```python
from build123d import *

# Parameters (mm, degrees)
SKETCH1_W               = 31.75
SKETCH1_H               = 31.75
BOSS_EXTRUDE1_DEPTH     = 3.175
SKETCH4_W               = 19.05
SKETCH4_H               = 19.05
BOSS_EXTRUDE2_DEPTH     = 9.525
F_5_8_11_TAPPED_HOLE2_D = 13.49248
CHAMFER1_SIZE           = 3.175


with BuildPart() as part:
    # Sketch1 → Boss-Extrude1 (new, symmetric)
    with BuildSketch(Plane.XY):
        Rectangle(SKETCH1_W, SKETCH1_H)
    extrude(amount=BOSS_EXTRUDE1_DEPTH, both=True)

    # Sketch4 → Boss-Extrude2 (add)
    with BuildSketch(Plane.XY.offset(3.175)):
        Rectangle(SKETCH4_W, SKETCH4_H)
    extrude(amount=BOSS_EXTRUDE2_DEPTH)

    # 5/8-11 Tapped Hole2 (through all)
    with Locations(Plane(origin=(0, 0, -3.175), x_dir=(-1, 0, 0), z_dir=(0, 0, -1))):
        with Locations((0, 0)):
            Hole(F_5_8_11_TAPPED_HOLE2_D / 2)

    # Chamfer1
    chamfer1_edges = [part.edges().sort_by_distance(p)[0] for p in [
        (-15.875, 15.875, 0),
        (15.875, 15.875, 0),
        (15.875, -15.875, 0),
        (-15.875, -15.875, 0),
    ]]
    chamfer(chamfer1_edges, length=CHAMFER1_SIZE)


solid = part.part
```
Build history of the part. All positions in model axes, mm. A direction names the side the tool comes from. Give positions to 0.01 mm unless a question says otherwise; leave off trailing zeros. Loops run counter-clockwise (first coordinate to the right, second up) from the corner with the lowest first, then second, coordinate; pieces in that order, holes last. Notation, with made-up numbers: (37, 64.5) -> (74, 64.5) arc R21 cw to (74, 97.5) -> close; hole circle Ø4 at (26.5, -11). An arc over 180 degrees is marked (long way). One line per question, with ' | ' between items. Start each with the question number.
1) Cut at C-C (z = 0.75). Give the cut face in (x, y) (3 decimals).
2) Cut at A-A (x = 0). Give the cut face in (y, z) (3 decimals).
3) Probe L1, parallel to Y at x = 0, z = 8 (3 decimals); L2, parallel to X at y = 7.5, z = 7.5 (3 decimals); L3, parallel to Z at x = 13, y = 14 (3 decimals). List the from-to ranges inside material, lowest first.
4) 3-axis set-ups, long thin cutter, end or side, ignore diameter. For faces 1 (the flat face through (0, 9.525, 8)), 2 (the flat face through (9.525, 0, 8)), 3 (the flat face through (-15.875, 0, 0)), 4 (the flat face through (-9.525, 0, 8)): which of +Z, -Z, +X, -X, +Y, -Y reach the whole face in a straight line?
5) Cut at D-D (z = 4.25). Give the cut face in (x, y) (3 decimals), plus the area to 3 significant figures.
6) Pin check, flat tips, straight feed: pin 1 (2 mm diameter, centred on y = -7, z = 10, fed in from -X) (3 decimals); pin 2 (4 mm diameter, centred on x = 9, y = 11, fed in from +Z); pin 3 (7.5 mm diameter, centred on y = -3.5, z = 9, fed in from +X) (3 decimals); pin 4 (8 mm diameter, centred on x = 0, y = 0, fed in from -Z). Stop position of each tip, or through.
7) Two-plate mould, pull along Y, no slides. Class faces 5 (the flat face through (0, -9.525, 8)), 6 (the flat face through (0, -10, 3.175)), 7 (the cylindrical face through (6.435, 2.026, 4.874)): released by +Y, released by -Y, zero draft, split by the parting line, or undercut.
Return value:
1) outline: (-15.875, -12.7) -> (-12.7, -15.875) -> (12.7, -15.875) -> (15.875, -12.7) -> (15.875, 12.7) -> (12.7, 15.875) -> (-12.7, 15.875) -> (-15.875, 12.7) -> close; hole circle Ø13.492 at (0, 0)
2) outline: (-15.875, -3.175) -> (-6.746, -3.175) -> (-6.746, 12.7) -> (-9.525, 12.7) -> (-9.525, 3.175) -> (-15.875, 3.175) -> close; (6.746, -3.175) -> (15.875, -3.175) -> (15.875, 3.175) -> (9.525, 3.175) -> (9.525, 12.7) -> (6.746, 12.7) -> close
3) L1: -9.525 to -6.746, 6.746 to 9.525 | L2: -9.525 to 9.525 | L3: -3.175 to 3.175
4) face 1: +Z, +X, -X, +Y | face 2: +Z, +X, +Y, -Y | face 3: +Z, -Z, -X, +Y, -Y | face 4: +Z, -X, +Y, -Y
5) outline: (-9.525, -9.525) -> (9.525, -9.525) -> (9.525, 9.525) -> (-9.525, 9.525) -> close; hole circle Ø13.492 at (0, 0) | area: 220 mm^2
6) pin 1: x = -9.525 | pin 2: z = 12.7 | pin 3: x = 9.525 | pin 4: through
7) face 5: released by -Y | face 6: zero draft | face 7: undercut
